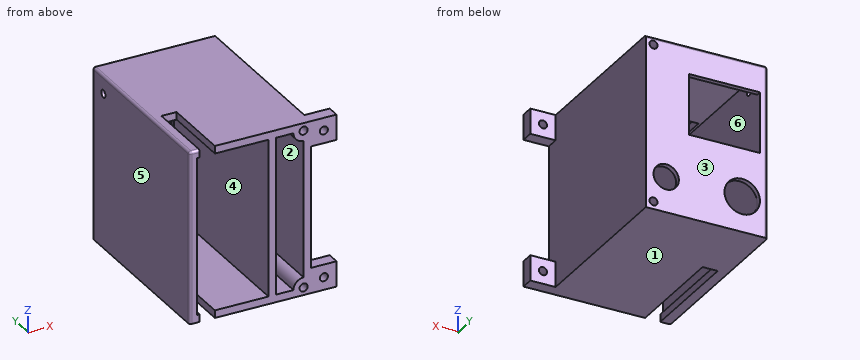
```python
from build123d import *

# Parameters (mm, degrees)
SKETCH1_W           = 48
SKETCH1_H           = 68
BOSS_EXTRUDE1_DEPTH = 71
SKETCH2_W           = 42
SKETCH2_H           = 62
CUT_EXTRUDE1_DEPTH  = 69
SKETCH3_R           = 7
SKETCH3_R_2         = 5
SKETCH3_W           = 28
SKETCH3_H           = 24
CUT_EXTRUDE2_DEPTH  = 3
SKETCH4_W           = 6
SKETCH4_H           = 42
CUT_EXTRUDE3_DEPTH  = 3
SKETCH5_W           = 6
SKETCH5_H           = 28
CUT_EXTRUDE4_DEPTH  = 3
SKETCH6_W           = 3
SKETCH6_H           = 62
BOSS_EXTRUDE2_DEPTH = 69
SKETCH7_R           = 1.5
CUT_EXTRUDE5_DEPTH  = 3
SKETCH11_R          = 1.6
BOSS_EXTRUDE3_DEPTH = 71
SKETCH12_R          = 1.6
CUT_EXTRUDE6_DEPTH  = 71
BOSS_EXTRUDE4_DEPTH = 71
SKETCH14_R          = 1.6
CUT_EXTRUDE7_DEPTH  = 71
FILLET2_R           = 1
FILLET3_R           = 1
FILLET5_R           = 1
SKETCH17_W          = 10
SKETCH17_H          = 5
BOSS_EXTRUDE5_DEPTH = 10
SKETCH18_R          = 1.6
CUT_EXTRUDE8_DEPTH  = 5
SKETCH19_W          = 10
SKETCH19_H          = 5
BOSS_EXTRUDE6_DEPTH = 10
SKETCH20_R          = 1.6
CUT_EXTRUDE10_DEPTH = 5


with BuildPart() as part:
    # Sketch1 → Boss-Extrude1 (new body)
    with BuildSketch(Plane(origin=(0, 0, 0), x_dir=(1, 0, 0), z_dir=(0, 1, 0))):
        with Locations((0.690647482, -20.618705036)):
            Rectangle(SKETCH1_W, SKETCH1_H)
    extrude(amount=BOSS_EXTRUDE1_DEPTH)

    # Sketch2 → Cut-Extrude1 (cut)
    with BuildSketch(Plane.XZ):
        with Locations((0.690647482, 20.618705036)):
            Rectangle(SKETCH2_W, SKETCH2_H)
    extrude(amount=-CUT_EXTRUDE1_DEPTH, mode=Mode.SUBTRACT)

    # Sketch3 → Cut-Extrude2 (cut)
    with BuildSketch(Plane(origin=(0, 71, 0), x_dir=(1, 0, 0), z_dir=(0, 1, 0))):
        with Locations((-13.309352518, -0.618705036)):
            Circle(SKETCH3_R)
        with Locations((16.690647482, -0.618705036)):
            Circle(SKETCH3_R_2)
        with Locations((-6.309352518, -31.618705036)):
            Rectangle(SKETCH3_W, SKETCH3_H)
    extrude(amount=-CUT_EXTRUDE2_DEPTH, mode=Mode.SUBTRACT)

    # Sketch4 → Cut-Extrude3 (cut)
    with BuildSketch(Plane(origin=(0, 0, -13.381294964), x_dir=(-1, 0, 0), z_dir=(0, 0, -1))):
        with Locations((16.309352518, 21)):
            Rectangle(SKETCH4_W, SKETCH4_H)
    extrude(amount=-CUT_EXTRUDE3_DEPTH, mode=Mode.SUBTRACT)

    # Sketch5 → Cut-Extrude4 (cut)
    with BuildSketch(Plane.XY.offset(54.618705036)):
        with Locations((-16.309352518, 14)):
            Rectangle(SKETCH5_W, SKETCH5_H)
    extrude(amount=-CUT_EXTRUDE4_DEPTH, mode=Mode.SUBTRACT)

    # Sketch6 → Boss-Extrude2 (add)
    with BuildSketch(Plane.XZ.offset(-69)):
        with Locations((9.33286699, 20.618705036)):
            Rectangle(SKETCH6_W, SKETCH6_H)
    extrude(amount=BOSS_EXTRUDE2_DEPTH)

    # Sketch7 → Cut-Extrude5 (cut)
    with BuildSketch(Plane.ZY.offset(23.309352518)):
        with Locations((47.618705036, 63)):
            Circle(SKETCH7_R)
    extrude(amount=-CUT_EXTRUDE5_DEPTH, mode=Mode.SUBTRACT)

    # Sketch11 → Boss-Extrude3 (add)
    with BuildSketch(Plane(origin=(0, 71, 0), x_dir=(1, 0, 0), z_dir=(0, 1, 0))):
        with BuildLine():
            Line((19.044896171, 13.381294964), (24.690647482, 13.381294964))
            Line((24.690647482, 13.381294964), (24.690647482, 7.735543653))
            ThreePointArc((24.690647482, 7.735543653), (18.862220357, 7.552867839), (19.044896171, 13.381294964))
        make_face()
        with Locations((21.690647482, 10.381294964)):
            Circle(SKETCH11_R, mode=Mode.SUBTRACT)
    extrude(amount=-BOSS_EXTRUDE3_DEPTH)

    # Sketch12 → Cut-Extrude6 (cut)
    with BuildSketch(Plane(origin=(0, 71, 0), x_dir=(1, 0, 0), z_dir=(0, 1, 0))):
        with Locations((21.690647482, 10.381294964)):
            Circle(SKETCH12_R)
    extrude(amount=-CUT_EXTRUDE6_DEPTH, mode=Mode.SUBTRACT)

    # Sketch13 → Boss-Extrude4 (add)
    with BuildSketch(Plane(origin=(0, 71, 0), x_dir=(1, 0, 0), z_dir=(0, 1, 0))):
        with BuildLine():
            Line((19.044896171, -54.618705036), (24.690647482, -54.618705036))
            Line((24.690647482, -54.618705036), (24.690647482, -48.972953725))
            ThreePointArc((24.690647482, -48.972953725), (18.862220357, -48.790277911), (19.044896171, -54.618705036))
        make_face()
    extrude(amount=-BOSS_EXTRUDE4_DEPTH)

    # Sketch14 → Cut-Extrude7 (cut)
    with BuildSketch(Plane(origin=(0, 71, 0), x_dir=(1, 0, 0), z_dir=(0, 1, 0))):
        with Locations((21.690647482, -51.618705036)):
            Circle(SKETCH14_R)
    extrude(amount=-CUT_EXTRUDE7_DEPTH, mode=Mode.SUBTRACT)

    # Fillet2
    fillet2_edges = [part.edges().sort_by_distance(p)[0] for p in [
        (0.690647482, 71, 54.618705036),
    ]]
    fillet(fillet2_edges, radius=FILLET2_R)

    # Fillet3
    fillet3_edges = [part.edges().sort_by_distance(p)[0] for p in [
        (-23.309352518, 35, 54.618705036),
        (-23.309352518, 70.707106781, 54.325811817),
        (-23.309352518, 71, 20.118705036),
    ]]
    fillet(fillet3_edges, radius=FILLET3_R)

    # Fillet5
    fillet5_edges = [part.edges().sort_by_distance(p)[0] for p in [
        (-20.809352518, 0, 54.618705036),
        (-23.016459299, 0, 54.325811817),
        (-23.309352518, 0, 20.118705036),
    ]]
    fillet(fillet5_edges, radius=FILLET5_R)

    # Sketch17 → Boss-Extrude5 (add)
    with BuildSketch(Plane(origin=(24.690647482, 0, 0), x_dir=(0, 0, -1), z_dir=(1, 0, 0))):
        with Locations((-49.618705036, 2.5)):
            Rectangle(SKETCH17_W, SKETCH17_H)
    extrude(amount=BOSS_EXTRUDE5_DEPTH)

    # Sketch18 → Cut-Extrude8 (cut)
    with BuildSketch(Plane(origin=(0, 5, 0), x_dir=(1, 0, 0), z_dir=(0, 1, 0))):
        with Locations((29.690647482, -49.618705036)):
            Circle(SKETCH18_R)
    extrude(amount=-CUT_EXTRUDE8_DEPTH, mode=Mode.SUBTRACT)

    # Sketch19 → Boss-Extrude6 (add)
    with BuildSketch(Plane(origin=(24.690647482, 0, 0), x_dir=(0, 0, -1), z_dir=(1, 0, 0))):
        with Locations((8.381294964, 2.5)):
            Rectangle(SKETCH19_W, SKETCH19_H)
    extrude(amount=BOSS_EXTRUDE6_DEPTH)

    # Sketch20 → Cut-Extrude10 (cut)
    with BuildSketch(Plane(origin=(0, 5, 0), x_dir=(1, 0, 0), z_dir=(0, 1, 0))):
        with Locations((29.690647482, 8.381294964)):
            Circle(SKETCH20_R)
    extrude(amount=-CUT_EXTRUDE10_DEPTH, mode=Mode.SUBTRACT)


solid = part.part
```
Source: CAD feature listing. Evaluate the final solid. Frame: model axes, mm. Face numbers are marked on the shaded views. A direction names the side the tool comes from. Coordinates: 2 decimals unless noted, no trailing zeros. Loops run counter-clockwise (first coordinate to the right, second up) from the corner with the lowest first, then second, coordinate; pieces in that order, holes last. Notation, with made-up numbers: M 34.5,61.5 L 41.5,61.5 A25 cw 41.5,90.5 Z; hole C 26,78 d1. An arc over 180 degrees is marked long. Use CSV: the item, a comma, the result in double quotes.
(1) Contact query for flat-ended pins moving along their axis: pin 1 (0.9 mm diameter, centred on x = -15, z = -12, fed in from -Y); pin 2 (8 mm diameter, centred on x = 29, z = 27.5, fed in from +Y); pin 3 (18.5 mm diameter, centred on y = 18, z = 32.5, fed in from +X). Output: stop coordinate, or through.
Answers follow:
pin 1,"y = 42"
pin 2,"through"
pin 3,"x = 24.69"
(2) Draft query along X for the marked faces 3, 4, 5 and 6. Return one class per face: pulls with the +X half, pulls with the -X half, needs draft (parallel to the pull), parting line crosses it, or undercut.
Answers follow:
face 3,"needs draft"
face 4,"undercut"
face 5,"pulls with the -X half"
face 6,"undercut"
(3) Cut plane C-C on z = 40. Return loops of the section in (x, y).
Answers follow:
outline,"M -23.31,1 A1 ccw -22.31,0 L -20.31,0 L -20.31,71 L -22.31,71 A1 ccw -23.31,70 Z; M 7.69,69 L 7.83,69 L 7.83,0 L 10.83,0 L 10.83,69 L 21.69,69 L 21.69,0 L 24.69,0 L 24.69,71 L 7.69,71 Z"
(4) Reachability of the marked faces 1 and 2 from +Z, -Z, +X, -X, +Y, -Y: full face, straight path, thin tool, end or side. Return the list, or none.
Answers follow:
face 1,"-Z, +X, -X, +Y, -Y"
face 2,"-Y"
(5) Line query: line 1 (X direction, y = 56.5, z = 3); line 2 (Z direction, x = -19, y = 43); line 3 (Y direction, x = 21, z = 21). Output: solid intervals per line, ascending. Write a range as [from, to].
Answers follow:
line 1,"[-23.31, -20.31], [7.83, 10.83], [21.69, 24.69]"
line 2,"[-13.38, -10.38], [51.62, 54.62]"
line 3,"[69, 71]"
(6) Cut plane B-B on y = 59.5. Return loops of the section in (x, z), and give its area (3 significant figures).
Answers follow:
outline,"M -23.31,-13.38 L 24.69,-13.38 L 24.69,54.62 L -22.31,54.62 A1 ccw -23.31,53.62 Z; hole M -20.31,-10.38 L 7.83,-10.38 L 7.83,51.62 L -20.31,51.62 Z; hole M 10.83,-10.38 L 17.69,-10.38 A4 cw 21.69,-6.38 L 21.69,47.62 A4 cw 17.69,51.62 L 10.83,51.62 Z; hole C 21.69,-10.38 d3.2; hole C 21.69,51.62 d3.2"
area,"855 mm²"
(7) Cut plane D-D on y = 31. Return loops of the section in (x, z).
Answers follow:
outline,"M -23.31,-13.38 L -19.31,-13.38 L -19.31,-10.38 L -20.31,-10.38 L -20.31,51.62 L 7.83,51.62 L 7.83,-10.38 L -13.31,-10.38 L -13.31,-13.38 L 24.69,-13.38 L 24.69,54.62 L -22.31,54.62 A1 ccw -23.31,53.62 Z; hole M 10.83,-10.38 L 17.69,-10.38 A4 cw 21.69,-6.38 L 21.69,47.62 A4 cw 17.69,51.62 L 10.83,51.62 Z; hole C 21.69,-10.38 d3.2; hole C 21.69,51.62 d3.2"
(8) Cut plane A-A on y = 20. Return loops of the section in (x, z).
Answers follow:
outline,"M -23.31,-13.38 L -19.31,-13.38 L -19.31,-10.38 L -20.31,-10.38 L -20.31,51.62 L -19.31,51.62 L -19.31,54.62 L -22.31,54.62 A1 ccw -23.31,53.62 Z; M -13.31,-13.38 L 24.69,-13.38 L 24.69,54.62 L -13.31,54.62 L -13.31,51.62 L 7.83,51.62 L 7.83,-10.38 L -13.31,-10.38 Z; hole M 10.83,-10.38 L 17.69,-10.38 A4 cw 21.69,-6.38 L 21.69,47.62 A4 cw 17.69,51.62 L 10.83,51.62 Z; hole C 21.69,-10.38 d3.2; hole C 21.69,51.62 d3.2"
